Work out the finished part from the listing and answer in its coordinate system (mm). Face numbers are marked on the shaded views. Coordinates: 2 decimals unless noted, no trailing zeros. Order: outer loops, then holes, each group sorted by start corner. A loop starts at its lowest first (then second) coordinate and runs counter-clockwise, first axis right, second up.
```python
from build123d import *

# Parameters (mm, degrees)
SKETCH1_R           = 2.75
SKETCH1_R_2         = 1
EXTRUDE_THIN1_DEPTH = 1.75
FILLET1_R           = 0.5
FILLET2_R           = 0.1
SCALE1_SCALE        = 10


with BuildPart() as part:
    # Sketch1 → Extrude-Thin1 (new body)
    with BuildSketch(Plane.XY):
        Circle(SKETCH1_R)
        Circle(SKETCH1_R_2, mode=Mode.SUBTRACT)
    extrude(amount=EXTRUDE_THIN1_DEPTH)

    # Fillet1
    fillet1_edges = [part.edges().sort_by_distance(p)[0] for p in [
        (-2.75, 0, 0),
    ]]
    fillet(fillet1_edges, radius=FILLET1_R)

    # Fillet2
    fillet2_edges = [part.edges().sort_by_distance(p)[0] for p in [
        (-1, 0, 0),
        (-2.75, 0, 1.75),
        (-1, 0, 1.75),
    ]]
    fillet(fillet2_edges, radius=FILLET2_R)


with BuildPart() as part_1:
    # Scale1: scaled about (0, 0, 0.893384529)
    add(part.part.scale(SCALE1_SCALE).moved(Location((0, 0, -8.040460761))))


solid = part_1.part
```
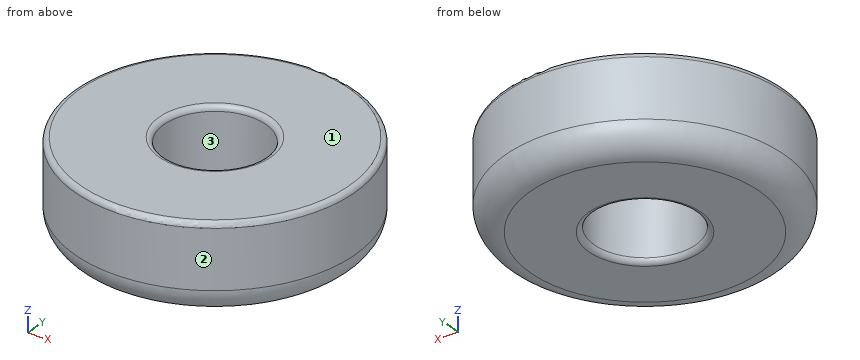
1. The mould has two halves that part along X. Classify the marked faces 1, 2 and 3: released by +X, released by -X, zero draft, split by the parting line, or undercut.
2. The part is cut by section C-C (z = 2.5). Determine the outline of the cut face in (x, y), plus the area to 3 significant figures.
3. The part is cut by section A-A (y = 0). Determine the outline of the cut face in (x, z).
4. Consider probe 1 along Y at (x, z) = (0, 2.5); probe 2 along X at (y, z) = (-3, 8); probe 3 along Y at (x, z) = (-5.5, -6.75). Determine where each line is inside the solid, lowest interval first.
5. Flat-ended cylindrical pins translate along their axes: pin 1 (1 mm diameter, centred on y = 7, z = -5.5, fed in from -X); pin 2 (1 mm diameter, centred on x = -5, z = -3, fed in from +Y); pin 3 (6 mm diameter, centred on x = 19, z = 5.5, fed in from -Y). Find the tip coordinate at first contact, or state that the pin passes through.
Worked out:
1. face 1: zero draft
1. face 2: split by the parting line
1. face 3: undercut
2. outline: circle Ø55 at (0, 0); hole circle Ø20 at (0, 0)
2. area: 2,060 mm2
3. outline: (-27.5, -3.04) arc R5 ccw to (-22.5, -8.04) - (-11, -8.04) arc R1 ccw to (-10, -7.04) - (-10, 8.46) arc R1 ccw to (-11, 9.46) - (-26.5, 9.46) arc R1 ccw to (-27.5, 8.46) - close; (10, -7.04) arc R1 ccw to (11, -8.04) - (22.5, -8.04) arc R5 ccw to (27.5, -3.04) - (27.5, 8.46) arc R1 ccw to (26.5, 9.46) - (11, 9.46) arc R1 ccw to (10, 8.46) - close
4. probe 1: y = -27.5 to -10, 10 to 27.5
4. probe 2: x = -27.34 to -9.54, 9.54 to 27.34
4. probe 3: y = -25.26 to -8.35, 8.35 to 25.26
5. pin 1: stops at x = -26.22
5. pin 2: stops at y = 27.13
5. pin 3: stops at y = -22.37
